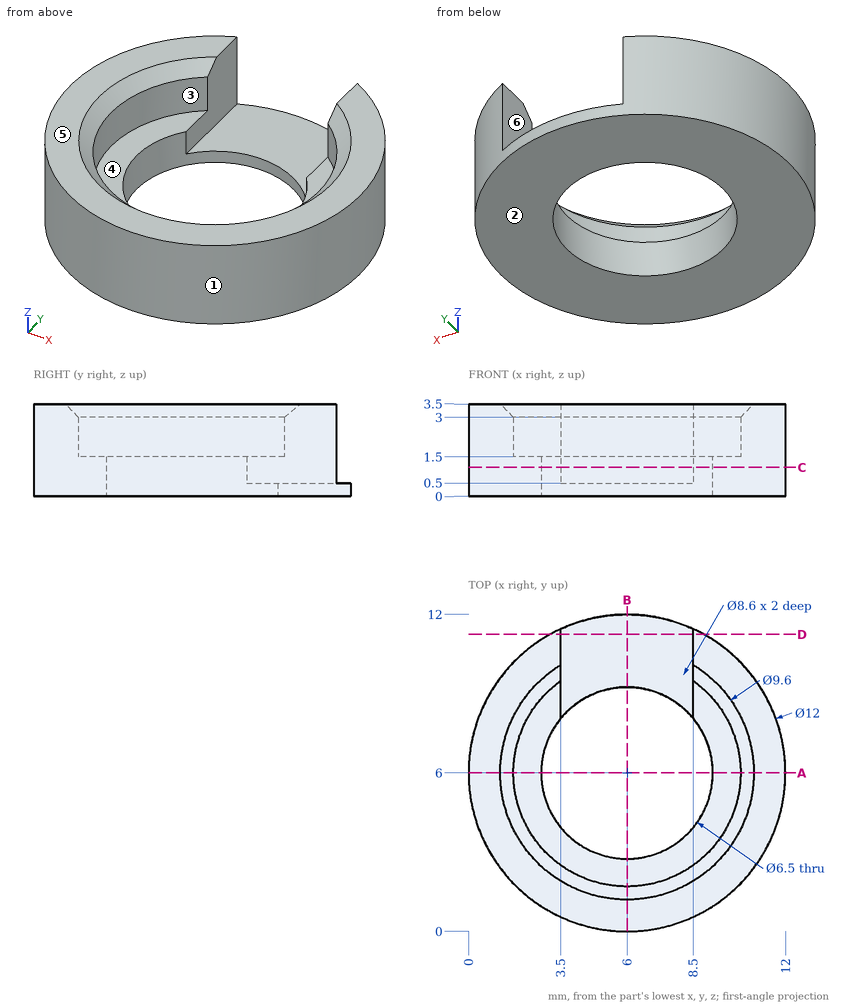
Print and shaded views of the part. All mm, measured from the part's lowest x, y and z. A direction names the side the tool comes from. Coordinates: 2 decimals unless noted, no trailing zeros. Order: outer loops, then holes, each group sorted by start corner. A loop starts at its lowest first (then second) coordinate and runs counter-clockwise, first axis right, second up. Notation, with made-up numbers: M 50.5,80.5 L 65.5,80.5 A17 cw 65.5,96.5 Z; hole C -28.5,68.25 d3. An arc over 180 degrees is marked long. Write each question's results on one line, items separated by ' | '. Start each with the question number.
Q1. Cut at C-C (z = 1.1). List the corners of the cut face in (x, y).
Q2. Pull direction Y, two halves, no side cores. Call the marked faces 1, 2 and 3: +Y half, -Y half, draft (parallel to the pull), parting line (faces both ways), or undercut.
Q3. Cut at B-B (x = 6). List the corners of the cut face in (y, z), then the cut area to 4 significant figures.
Q4. Cut at A-A (y = 6). List the corners of the cut face in (x, z), then the cut area to 3 significant figures.
Q5. Cut at D-D (y = 11.25). List the corners of the cut face in (x, z), then the cut area to 3 significant figures.
Q6. Flat gauge pin, fed straight in: P1, Ø1.5, axis at y = 10, z = 2, coming from the +X side. Where does the tip first touch, or does it go through?
Q7. Which spindle directions (+Z, -Z, +X, -X, +Y, -Y) get a long thin tool onto all of the face, cutting with end or side? Do the marked faces 4, 5 and 6. Say none if no direction does.
Q8. Drill centre lines: probe 1 along X at (y, z) = (6, 2.15); probe 2 along X at (y, z) = (6, 0.5); probe 3 along Y at (x, z) = (2.75, 1.8). Where is each one in solid material? Low to high. Write a range as from..to.
Found:
1) outline: M 3.5,8.08 L 3.5,11.45 A6 ccw long 8.5,11.45 L 8.5,8.08 A3.25 cw long Z
2) face 1: parting line | face 2: draft | face 3: undercut
3) outline: M 0,0 L 2.75,0 L 2.75,1.5 L 1.7,1.5 L 1.7,3 L 1.2,3.5 L 0,3.5 Z; M 9.25,0 L 12,0 L 12,0.5 L 9.25,0.5 Z | area: 8.775 mm²
4) outline: M 0,0 L 2.75,0 L 2.75,1.5 L 1.7,1.5 L 1.7,3 L 1.2,3.5 L 0,3.5 Z; M 9.25,0 L 12,0 L 12,3.5 L 10.8,3.5 L 10.3,3 L 10.3,1.5 L 9.25,1.5 Z | area: 14.8 mm²
5) outline: M 3.1,0 L 8.9,0 L 8.9,3.5 L 8.5,3.5 L 8.5,0.5 L 3.5,0.5 L 3.5,3.5 L 3.1,3.5 Z | area: 5.33 mm²
6) P1: x = 11.04
7) face 4: +Z | face 5: +Z, +X, -X, +Y, -Y | face 6: +Z, +Y
8) probe 1: 0..1.7, 10.3..12 | probe 2: 0..2.75, 9.25..12 | probe 3: 0.96..3.18, 8.82..11.04
